The model under review builds one solid part; all positions refer to its coordinate system, in mm. Face numbers are marked on the shaded views. A direction names the side the tool comes from. Coordinates: 2 decimals unless noted, no trailing zeros. Write each loop counter-clockwise with the first axis right and the second up, starting at its lowest first coordinate (ties: lowest second). Pieces come first, ordered by that corner, then holes. Notation, with made-up numbers: (-25.5, 89) - (7.5, 89) arc R28 cw to (7.5, 112) - close; hole circle Ø4 at (75.5, 35). An arc over 180 degrees is marked (long way). Return JSON: item names as keys, results as strings. Group by question number.
(1) Tool access review of the marked faces 4 and 5: name each direction out of +Z, -Z, +X, -X, +Y, -Y from which nothing blocks a thin tool from reaching the whole face with its end or side.
(2) We need section C-C on y = 19. State the section outline as (x, z) points.
(3) We need section B-B on x = 26. State the section outline as (y, z) points, then the cut area to 3 significant figures.
(4) Draft analysis for pull direction Z (two halves, no side actions). For the marked faces 1, 2 and 3, state which applies: released by +Z, released by -Z, zero draft, split by the parting line, or undercut.
(5) To check wall thickness, follow L1, parallel to Z at x = 29.5, y = 4; L2, parallel to X at y = 26, z = -13; L3, parallel to Z at x = 19, y = 53. State the ranges of each line that lie inside material, in increasing order. Write a range as from..to.
(6) We need section A-A on z = -23. State the section outline as (x, y) points, then the cut area to 3 significant figures.
(7) We need section D-D on z = -2.5. State the section outline as (x, y) points, then the cut area to 3 significant figures.
(8) For pin 1 Ø8 at (x, z) = (1, -26.5) entering from -Y; pin 2 Ø0.8 at (x, y) = (31, 22.5) entering from +Z; pin 3 Ø3 at (x, z) = (17, 1.5) entering from +Y; pin 4 Ø4 at (x, y) = (7, 19) entering from +Z, all flat-tipped, find the tip position at first contact; note any pin that passes through.
```python
from build123d import *

# Parameters (mm, degrees)
SKETCH1_W           = 35
SKETCH1_H           = 35
SKETCH1_W_2         = 30
SKETCH1_H_2         = 30
BOSS_EXTRUDE1_DEPTH = 70
SKETCH2_W           = 17
SKETCH2_H           = 20
CUT_EXTRUDE1_DEPTH  = 2.5
CUT_EXTRUDE2_DEPTH  = 36


with BuildPart() as part:
    # Sketch1 → Boss-Extrude1 (new body)
    with BuildSketch(Plane(origin=(0, 0, 0), x_dir=(1, 0, 0), z_dir=(0, 1, 0))):
        with Locations((15, 15)):
            Rectangle(SKETCH1_W, SKETCH1_H)
        with Locations((15, 15)):
            Rectangle(SKETCH1_W_2, SKETCH1_H_2, mode=Mode.SUBTRACT)
    extrude(amount=BOSS_EXTRUDE1_DEPTH)

    # Sketch2 → Cut-Extrude1 (cut)
    with BuildSketch(Plane.XY.offset(2.5)):
        with Locations((15, 60)):
            Rectangle(SKETCH2_W, SKETCH2_H)
    extrude(amount=-CUT_EXTRUDE1_DEPTH, mode=Mode.SUBTRACT)

    # Sketch3 → Cut-Extrude2 (cut, through all)
    with BuildSketch(Plane.ZY.offset(2.5)):
        Polygon((2.5, 33), (-13.583801904, 25.5), (-13.583801904, 14.5), (2.5, 7), align=None)
    extrude(amount=-CUT_EXTRUDE2_DEPTH, mode=Mode.SUBTRACT)


solid = part.part
```
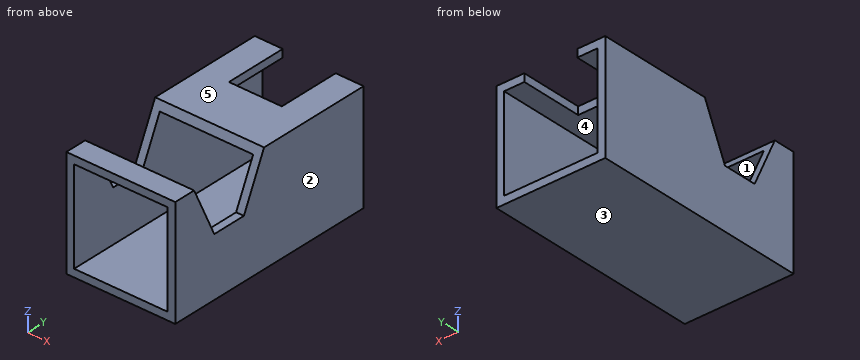
Ans:
{
 "1": {"face 4": "+Y, -Y", "face 5": "+Z, +X, -X, +Y, -Y"},
 "2": {"outline": "(-2.5, -32.5) - (32.5, -32.5) - (32.5, -13.58) - (30, -13.58) - (30, -30) - (0, -30) - (0, -13.58) - (-2.5, -13.58) - close"},
 "3": {"outline": "(0, -32.5) - (70, -32.5) - (70, -30) - (0, -30) - close; (0, 0) - (8.17, 0) - (7, 2.5) - (0, 2.5) - close; (31.83, 0) - (70, 0) - (70, 2.5) - (33, 2.5) - close", "area": "288 mm²"},
 "4": {"face 1": "undercut", "face 2": "zero draft", "face 3": "released by -Z"},
 "5": {"L1": "-32.5..-30, 0..2.5", "L2": "-2.5..0, 30..32.5", "L3": "-32.5..-30"},
 "6": {"outline": "(-2.5, 0) - (0, 0) - (0, 70) - (-2.5, 70) - close; (30, 0) - (32.5, 0) - (32.5, 70) - (30, 70) - close", "area": "350 mm²"},
 "7": {"outline": "(-2.5, 0) - (0, 0) - (0, 9.33) - (-2.5, 9.33) - close; (-2.5, 30.67) - (0, 30.67) - (0, 70) - (-2.5, 70) - close; (30, 0) - (32.5, 0) - (32.5, 9.33) - (30, 9.33) - close; (30, 30.67) - (32.5, 30.67) - (32.5, 70) - (30, 70) - close", "area": "243 mm²"},
 "8": {"pin 1": "y = 0", "pin 2": "z = -13.58", "pin 3": "y = 50", "pin 4": "z = -30"}
}
